from build123d import *

# Parameters (mm, degrees)
SKIZZE1_W                       = 24
SKIZZE1_H                       = 30
AUFSATZ_LINEAR_AUSTRAGEN1_DEPTH = 3
SKIZZE2_R                       = 10.5
SCHNITT_LINEAR_AUSTRAGEN2_DEPTH = 5
SKIZZE2_3_R                     = 9
SCHNITT_LINEAR_AUSTRAGEN3_DEPTH = 7
VERRUNDUNG1_R                   = 3
M3_GEWINDEBOHRUNG1_D            = 2.5
M3_GEWINDEBOHRUNG1_DEPTH        = 7
M3_GEWINDEBOHRUNG1_TIP          = 0.751075774


with BuildPart() as part:
    # Skizze1 → Aufsatz-Linear austragen1 (new body, symmetric)
    with BuildSketch(Plane.XY):
        with Locations((0, 15)):
            Rectangle(SKIZZE1_W, SKIZZE1_H)
    extrude(amount=AUFSATZ_LINEAR_AUSTRAGEN1_DEPTH, both=True)

    # Skizze2 → Schnitt-Linear austragen2 (cut)
    with BuildSketch(Plane.XY.offset(3)):
        with Locations((0, 15.5)):
            Circle(SKIZZE2_R)
    extrude(amount=-SCHNITT_LINEAR_AUSTRAGEN2_DEPTH, mode=Mode.SUBTRACT)

    # Skizze2<3> → Schnitt-Linear austragen3 (cut, through all)
    with BuildSketch(Plane.XY.offset(3)):
        with Locations((0, 15.5)):
            Circle(SKIZZE2_3_R)
    extrude(amount=-SCHNITT_LINEAR_AUSTRAGEN3_DEPTH, mode=Mode.SUBTRACT)

    # Verrundung1
    verrundung1_edges = [part.edges().sort_by_distance(p)[0] for p in [
        (-12, 30, 0),
        (12, 30, 0),
    ]]
    fillet(verrundung1_edges, radius=VERRUNDUNG1_R)

    # M3 Gewindebohrung1
    with Locations(Plane(origin=(0, 0, 0), x_dir=(-1, 0, 0), z_dir=(0, -1, 0))):
        with Locations((-7, -0.5), (7, -0.5)):
            Hole(M3_GEWINDEBOHRUNG1_D / 2, depth=M3_GEWINDEBOHRUNG1_DEPTH)
            with Locations((0, 0, -(M3_GEWINDEBOHRUNG1_DEPTH + M3_GEWINDEBOHRUNG1_TIP / 2))):  # 118° drill point
                Cone(0, M3_GEWINDEBOHRUNG1_D / 2, M3_GEWINDEBOHRUNG1_TIP, mode=Mode.SUBTRACT)


solid = part.part
Here's how the part is built. I have some questions about the finished solid (model axes, mm). A direction names the side the tool comes from. Coordinates: 2 decimals unless noted, no trailing zeros. Order: outer loops, then holes, each group sorted by start corner. A loop starts at its lowest first (then second) coordinate and runs counter-clockwise, first axis right, second up. Notation, with made-up numbers: M -11.5,19.5 L 3.5,19.5 A26 ccw 3.5,54.5 Z; hole C 6.25,53.5 d4. An arc over 180 degrees is marked long. Answer as CSV lines item,"result".
Item 1: On a 3-axis mill with a long thin cutter (end or side, diameter ignored), from which of +Z, -Z, +X, -X, +Y, -Y can I reach the whole of each face in a straight line? I mean faces 1 (the face through (8, 20, -2)), 2 (the face through (5.75, 3.55, 0.45)), 3 (the face through (12, 13, 0)). Say none if no direction works.
Results found:
face 1,"+Z"
face 2,"-Y"
face 3,"+Z, -Z, +X, +Y, -Y"
Item 2: Imagine slicing it at C-C on z = 0.5. Write out the boundary of the cut face in (x, y), plus the area to 3 significant figures.
Results found:
outline,"M -12,0 L -8.25,0 L -8.25,7 L -7.05,7.72 A10.5 cw long 7.05,7.72 L 8.25,7 L 8.25,0 L 12,0 L 12,27 A3 ccw 9,30 L -9,30 A3 ccw -12,27 Z; M -5.75,0 L 5.75,0 L 5.75,6.71 A10.5 cw -5.75,6.71 Z"
area,"333 mm2"
Item 3: Imagine slicing it at B-B on y = 15.5. Write out the boundary of the cut face in (x, z).
Results found:
outline,"M -12,-3 L -9,-3 L -9,-2 L -10.5,-2 L -10.5,3 L -12,3 Z; M 9,-3 L 12,-3 L 12,3 L 10.5,3 L 10.5,-2 L 9,-2 Z"
Item 4: For pin 1 (3 mm diameter, centred on x = -3, z = 2.5, fed in from -Y); pin 2 (5 mm diameter, centred on x = 4.5, y = 9, fed in from +Z), each with a flat end and sliding along its axis, tell me the tip position at first contact or that it passes through.
Results found:
pin 1,"y = 0"
pin 2,"z = -2"
Item 5: Imagine slicing it at A-A on x = 0. Write out the boundary of the cut face in (y, z).
Results found:
outline,"M 0,-3 L 6.5,-3 L 6.5,-2 L 5,-2 L 5,3 L 0,3 Z; M 24.5,-3 L 30,-3 L 30,3 L 26,3 L 26,-2 L 24.5,-2 Z"
Item 6: If I drill on line 1 (Y direction, x = 0, z = -2.6); line 2 (Y direction, x = 0, z = -1); line 3 (Z direction, x = 7, y = 2.25), over which ranges is the centre line in solid material (lowest first)?
Results found:
line 1,"0 to 6.5, 24.5 to 30"
line 2,"0 to 5, 26 to 30"
line 3,"-3 to -0.75, 1.75 to 3"
Item 7: We'd pull the mould along Z, two halves only. Please class faces 4 (the face through (0, 5, -3)), 5 (the face through (-12, 13, 0)), 6 (the face through (-7.393, 7.515, 0.513)): +Z half, -Z half, draft (parallel to the pull), parting line (faces both ways), or undercut.
Results found:
face 4,"-Z half"
face 5,"draft"
face 6,"undercut"
